Geometry: final body of the model. Coordinates: model frame, mm. Face numbers are marked on the shaded views. A direction names the side the tool comes from. Give positions to 0.01 mm unless a question says otherwise; leave off trailing zeros. Loops run counter-clockwise (first coordinate to the right, second up) from the corner with the lowest first, then second, coordinate; pieces in that order, holes last. Notation, with made-up numbers: (36, -24) - (69, -24) arc R7 cw to (69, -19) - close; hole circle Ø4 at (5, 72). An arc over 180 degrees is marked (long way). Use one line per item in the form item = value.
Autodesk Inventor part; units mm, degrees
ref_plane "YZ Plane" through (0, 0, 0) normal (1, 0, 0) x (0, 1, 0)
ref_plane "XZ Plane" through (0, 0, 0) normal (0, 1, 0) x (-1, 0, 0)
ref_plane "XY Plane" through (0, 0, 0) normal (0, 0, 1) x (1, 0, 0)
sketch "Sketch1" plane through (0, 0, 0) normal (1, 0, 0) x (0, 1, 0)
  line L0 (-0.54, 0) -> (-0.54, -14.29)
  circle A0 centre (-0.54, 0) radius 7.65
  line L1 (-0.54, -14.29) -> (14.79, -14.29)
  line L2 (14.79, -14.29) -> (-24.27, -14.29)
  line L3 (-24.27, -14.29) -> (-24.27, 14.29)
  line L4 (-24.27, 14.29) -> (14.79, 14.29)
  line L5 (14.79, 14.29) -> (14.79, -14.29)
  circle A1 centre (-0.54, 0) radius 16.22
  circle A2 centre (-0.54, 0) radius 23.01
  line L6 (-0.54, 0) -> (-0.54, -23.01)
  line L7 (-0.54, -23.01) -> (-0.54, -24.49)
  line L8 (-0.54, -23.01) -> (0.895, -23.01)
  ellipse E0 centre (-0.54, -23.01) end of major axis (-0.54, -24.49) minor radius 1.435
  circle A3 centre (-0.54, -16.22) radius 1.5
  line L9 (-8.19, 0) -> (-16.76, 0)
  line L10 (-8.19, 0) -> (-8.19, -14.29)
  line L11 (-0.54, -23.01) -> (-3.41, -23.01)
  circle A4 centre (-0.54, -23.01) radius 2.87
  line L12 (-8.19, -14.29) -> (-3.0986, -24.3101)
  line L13 (7.11, -14.29) -> (2.0186, -24.3101)
  ellipse E1 centre (-0.54, 23.01) end of major axis (-0.54, 24.49) minor radius 1.435
  circle A5 centre (-0.54, 16.22) radius 1.5
  circle A6 centre (-0.54, 23.01) radius 2.87
  line L14 (-8.19, 14.29) -> (-3.0986, 24.3101)
  line L15 (7.11, 14.29) -> (2.0186, 24.3101)
  point P0 (-3.4044, -22.831)
  point P1 (-1.9743, -22.9653)
  point P2 (-1.975, -23.01)
  point P3 (-8.1812, -14.3074)
  point P4 (-8.1812, 14.3074)
  point P5 (-8.2136, 14.29)
  point P6 (-8.2136, -14.29)
  dimension "d13" = 15.3
  dimension "d18" = 46.02
  dimension "d12" = 14.29
  dimension "d14" = 15.33
  dimension "d15" = 39.06
  dimension "d16" = 28.58
  dimension "d17" = 32.44
  dimension "d19" = 1.48
  dimension "d20" = 1.435
  dimension "d21" = 3
  dimension "d22" = 2.87
extrude "Extrusion1" add sketch "Sketch1" along normal blind 10.3 contours A0 L9 A1 L4 L5 L1 L0 | L0 L2 L10 A0 | L6 A3 A1 L12 L2 | L1 L13 A1 A3 L6 | L10 L2 A1 L9 | L12 A1 L2 | A1 L2 A2 L4 | A1 L5 L1 | L13 A2 A4 L6 A3 A1 | A1 A3 L6 A4 A2 L12 | A1 L14 L4 | L13 A4 A2 | L2 L3 L4 A2 | A2 A4 L12 | L14 A1 A5 L15 L4 | L14 A2 A6 L15 A1 A5 | A1 L4 L5 | A4 L11 E0 A2 | A2 E0 L6 A4 | A4 L6 E0 A2 | A2 E0 L11 A4 | L14 A6 A2 | A2 A6 L15 | A6 A2 E1 | A2 E1 A6
fillet "Fillet1" radius 15.49 2 edges at (5.15, 14.79, -14.29) (5.15, 14.79, 14.29)
chamfer "Chamfer1" distance 5 angle 45 2 edges at (5.15, -24.27, -14.29) (5.15, -24.27, 14.29)
sketch "Sketch2" plane through (10.3, 0, 0) normal (1, 0, 0) x (0, 0, -1)
  circle A0 centre (0, -0.54) radius 7.65
  line L0 (0, -0.54) -> (7.65, -0.54)
  circle A1 centre (0, -0.54) radius 4
  circle A2 centre (0, -0.54) radius 7.65
  point P0 (0, 0)
  dimension "d29" = 8
extrude "8mm_inlet" add sketch "Sketch2" against normal up to surface (10.3 mm away)
properties part number "AMT102-0512-I5000-5"
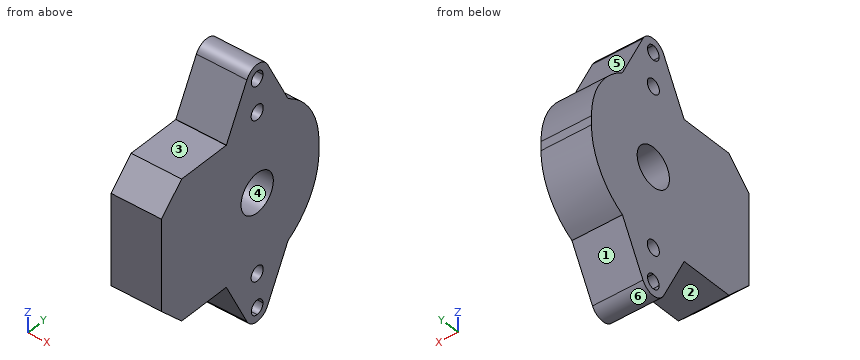
(1) Pull-direction query (Y, two-part tool) for the marked faces 4, 5 and 6; classes: released by +Y, released by -Y, zero draft, split by the parting line, or undercut.
Solution:
face_4 = undercut
face_5 = released by +Y
face_6 = split by the parting line
(2) Cut plane B-B (y = -16). Return the cut outline in (x, z), plus the area to 3 significant figures.
Solution:
outline = (0, -14.29) - (10.3, -14.29) - (10.3, 14.29) - (0, 14.29) - close
area = 294 mm2
(3) Material intervals for L1, parallel to Y at x = 4, z = 0; L2, parallel to Z at x = 3, y = -17; L3, parallel to Y at x = 6.5, z = 16.22, sorted ascending. Write a range as from..to.
Solution:
L1 = -24.27..-4.54, 3.46..14.79
L2 = -14.29..14.29
L3 = -7.21..-2.04, 0.96..6.13
(4) Cut plane A-A (z = 0). Return the cut outline in (x, y), plus the area to 3 significant figures.
Solution:
outline = (0, -24.27) - (10.3, -24.27) - (10.3, -4.54) - (0, -4.54) - close; (0, 3.46) - (10.3, 3.46) - (10.3, 14.79) - (0, 14.79) - close
area = 320 mm2
(5) Access query for the marked faces 1, 2 and 3. Directions: +Z, -Z, +X, -X, +Y, -Y. A direction counts if a zero-diameter tool reaches every point of the face in a straight line with its end or side. Return the directions, or none.
Solution:
face_1 = -Z, +X, -X, +Y
face_2 = -Z, +X, -X, -Y
face_3 = +Z, +X, -X, -Y
(6) Pin query (flat end, axial travel): P1, Ø4, axis at y = -9, z = -20.5, coming from the -X side; P2, Ø5, axis at x = 5, y = -4, coming from the -Z side; P3, Ø6, axis at x = 6, z = 15, coming from the +Y side; P4, Ø5, axis at x = 5.5, z = 12, coming from the +Y side. Return the tip coordinate at first contact, or that it passes through.
Solution:
P1 = through
P2 = -25.71
P3 = 10.12
P4 = 12.19
(7) Cut plane C-C (x = 5). Give the number of separate pieces and of enclosed holes in the cut face, plus the area to 3 significant figures.
Solution:
separate_pieces = 1
enclosed_holes = 5
area = 1,170 mm2
(8) Cut plane D-D (z = -16.22). Return the cut outline in (x, y), plus the area to 3 significant figures.
Solution:
outline = (0, -7.21) - (10.3, -7.21) - (10.3, -2.04) - (0, -2.04) - close; (0, 0.96) - (10.3, 0.96) - (10.3, 6.13) - (0, 6.13) - close
area = 106 mm2
